Geometry: final body of the model. Coordinates: model frame, mm. A direction names the side the tool comes from. Coordinates: 2 decimals unless noted, no trailing zeros. Loops run counter-clockwise (first coordinate to the right, second up) from the corner with the lowest first, then second, coordinate; pieces in that order, holes last. Notation, with made-up numbers: (-25.5, 29.5) - (24.5, 29.5) arc R18 cw to (24.5, 52.5) - close; hole circle Ø7 at (-36.5, 52.5). An arc over 180 degrees is marked (long way). Answer in a Markdown table with one row per item.
from build123d import *

# Parameters (mm, degrees)
BOSS_EXTRUDE1_DEPTH = 5.08
SKETCH2_3_R         = 1.45
CUT_EXTRUDE1_DEPTH  = 6.08


with BuildPart() as part:
    # Sketch2 → Boss-Extrude1 (new body)
    with BuildSketch(Plane.XY):
        Polygon((5.132895747, 7.719827316), (-5.755840057, 7.267231781), (-8.690200536, -3.228431071), (0.385000757, -9.262511914), (8.928144089, -2.496116113), align=None)
        Polygon((-8.928144089, 2.496116113), (-5.132895747, -7.719827316), (5.755840057, -7.267231781), (8.690200536, 3.228431071), (-0.385000757, 9.262511914), align=None)
    extrude(amount=BOSS_EXTRUDE1_DEPTH)

    # Sketch2_3 → Cut-Extrude1 (cut, through all)
    with BuildSketch(Plane.XY):
        Circle(SKETCH2_3_R)
    extrude(amount=CUT_EXTRUDE1_DEPTH, mode=Mode.SUBTRACT)


solid = part.part
(1) Access query for faces 4 (the face through (-8.41, 1.1, 2.5)), 5 (the face through (8.28, 1.76, 2.5)), 6 (the face through (3.65, 7.66, 2.5)). Directions: +Z, -Z, +X, -X, +Y, -Y. A direction counts if a zero-diameter tool reaches every point of the face in a straight line with its end or side. Return the directions, or none.
Verdict:
| item | result |
|---|---|
| face 4 | +Z, -Z, -X |
| face 5 | +Z, -Z, +X |
| face 6 | +Z, -Z, +Y |
(2) Cut plane A-A on y = -1. Output: boundary loops of the cut face in (x, z), then the cut area to 3 significant figures.
Verdict:
| item | result |
|---|---|
| outline | (-8.07, 0) - (-1.05, 0) - (-1.05, 5.08) - (-8.07, 5.08) - close; (1.05, 0) - (8.37, 0) - (8.37, 5.08) - (1.05, 5.08) - close |
| area | 72.8 mm² |
(3) Pull-direction query (Y, two-part tool) for faces 1 (the face through (4.23, -7.33, 2.5)), 2 (the face through (7.454, 4.051, 2.504)), 3 (the face through (8.41, -1.1, 2.5)); classes: pulls with the +Y half, pulls with the -Y half, needs draft (parallel to the pull), parting line crosses it, or undercut.
Verdict:
| item | result |
|---|---|
| face 1 | pulls with the -Y half |
| face 2 | pulls with the +Y half |
| face 3 | undercut |
(4) Cut plane D-D on y = 2.75. Output: boundary loops of the cut face in (x, z).
Verdict:
| item | result |
|---|---|
| outline | (-8.61, 0) - (8.56, 0) - (8.56, 5.08) - (-8.61, 5.08) - close |
(5) First-contact query: pin 1 Ø3 at (y, z) = (-2, 2) entering from -X; pin 2 Ø2.5 at (x, y) = (0, 0) entering from +Z; pin 3 Ø2 at (x, z) = (4, 3.5) entering from -Y; pin 4 Ø1.5 at (x, z) = (-5, 0.5) entering from +Y. Flat tips, straight axial feed; report the tip coordinate or a pass-through.
Verdict:
| item | result |
|---|---|
| pin 1 | stops at x = -8.69 |
| pin 2 | passes through |
| pin 3 | stops at y = -7.38 |
| pin 4 | stops at y = 7.33 |
(6) Ray query, probe 1 along Y at (x, z) = (0, 1.8); probe 2 along X at (y, z) = (0, 3.95); probe 3 along Y at (x, z) = (-0.5, 2.8). Return the intervals inside material, ascending.
Verdict:
| item | result |
|---|---|
| probe 1 | y = -9.01 to -1.45, 1.45 to 9.01 |
| probe 2 | x = -8 to -1.45, 1.45 to 8 |
| probe 3 | y = -8.67 to -1.36, 1.36 to 9.17 |
(7) Cut plane C-C on x = 0. Output: boundary loops of the cut face in (y, z), then the cut area to 3 significant figures.
Verdict:
| item | result |
|---|---|
| outline | (-9.01, 0) - (-1.45, 0) - (-1.45, 5.08) - (-9.01, 5.08) - close; (1.45, 0) - (9.01, 0) - (9.01, 5.08) - (1.45, 5.08) - close |
| area | 76.8 mm² |
